Source: CAD feature listing. Evaluate the final solid. Frame: model axes, mm. Coordinates: 2 decimals unless noted, no trailing zeros. Order: outer loops, then holes, each group sorted by start corner. A loop starts at its lowest first (then second) coordinate and runs counter-clockwise, first axis right, second up.
Item 1: Ray query, line 1 (Y direction, x = 0, z = 3.6); line 2 (X direction, y = 67.5, z = 0.2); line 3 (X direction, y = -4.5, z = 2.15). Return the intervals inside material, ascending.
Item 2: Section D-D on z = 3.3. Return the cut outline in (x, y).
Item 3: Section B-B on x = -50. Return the cut outline in (y, z).
Item 4: Section A-A on y = 27.6. Return the cut outline in (x, z), then the cut area to 3 significant figures.
Item 5: Section C-C on x = 0. Return the cut outline in (y, z).
Item 6: Contact query for flat-ended pins moving along their axis: P1, Ø4, axis at x = 0, y = 27.6, coming from the +Z side; P2, Ø1.5, axis at y = 45.5, z = 2.5, coming from the -X side; P3, Ø2.5, axis at y = 9.5, z = 2, coming from the +X side. Output: stop coordinate, or through.
from build123d import *

# Parameters (mm, degrees)
SKETCH1_W           = 20
SKETCH1_H           = 160
SKETCH1_H_2         = 40
SKETCH1_W_2         = 70
BOSS_EXTRUDE1_DEPTH = 5
SKETCH2_R           = 2.25
CUT_EXTRUDE1_DEPTH  = 15


with BuildPart() as part:
    # Sketch1 → Boss-Extrude1 (new body)
    with BuildSketch(Plane.XY):
        with Locations((0, 20)):
            Rectangle(SKETCH1_W, SKETCH1_H)
        with Locations((0, -80)):
            Rectangle(SKETCH1_W, SKETCH1_H_2)
        with Locations((-45, -80)):
            Rectangle(SKETCH1_W_2, SKETCH1_H_2)
        with Locations((45, -80)):
            Rectangle(SKETCH1_W_2, SKETCH1_H_2)
    extrude(amount=BOSS_EXTRUDE1_DEPTH)

    # Sketch2 → Cut-Extrude1 (cut)
    with BuildSketch(Plane.XY.offset(5)):
        with Locations((0, -91.6)):
            Circle(SKETCH2_R)
        with Locations((-50, -76)):
            Circle(SKETCH2_R)
        with Locations((50, -76)):
            Circle(SKETCH2_R)
        with Locations((0, 27.6)):
            Circle(SKETCH2_R)
        with Locations((0, 67.6)):
            Circle(SKETCH2_R)
        with Locations((0, -32.4)):
            Circle(SKETCH2_R)
        with Locations((0, -61.6)):
            Circle(SKETCH2_R)
    extrude(amount=-CUT_EXTRUDE1_DEPTH, mode=Mode.SUBTRACT)


solid = part.part
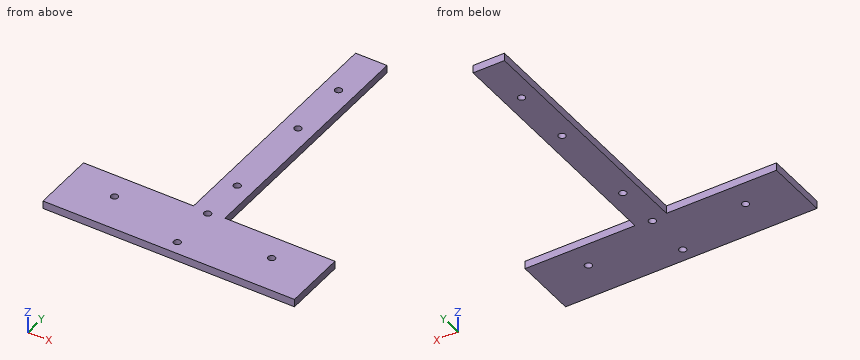
Answer list:
1. line 1: y = -100 to -93.85, -89.35 to -63.85, -59.35 to -34.65, -30.15 to 25.35, 29.85 to 65.35, 69.85 to 100
1. line 2: x = -10 to -2.25, 2.25 to 10
1. line 3: x = -10 to 10
2. outline: (-80, -100) - (80, -100) - (80, -60) - (10, -60) - (10, 100) - (-10, 100) - (-10, -60) - (-80, -60) - close; hole circle Ø4.5 at (-50, -76); hole circle Ø4.5 at (0, -91.6); hole circle Ø4.5 at (0, -61.6); hole circle Ø4.5 at (0, -32.4); hole circle Ø4.5 at (0, 27.6); hole circle Ø4.5 at (0, 67.6); hole circle Ø4.5 at (50, -76)
3. outline: (-100, 0) - (-78.25, 0) - (-78.25, 5) - (-100, 5) - close; (-73.75, 0) - (-60, 0) - (-60, 5) - (-73.75, 5) - close
4. outline: (-10, 0) - (-2.25, 0) - (-2.25, 5) - (-10, 5) - close; (2.25, 0) - (10, 0) - (10, 5) - (2.25, 5) - close
4. area: 77.5 mm2
5. outline: (-100, 0) - (-93.85, 0) - (-93.85, 5) - (-100, 5) - close; (-89.35, 0) - (-63.85, 0) - (-63.85, 5) - (-89.35, 5) - close; (-59.35, 0) - (-34.65, 0) - (-34.65, 5) - (-59.35, 5) - close; (-30.15, 0) - (25.35, 0) - (25.35, 5) - (-30.15, 5) - close; (29.85, 0) - (65.35, 0) - (65.35, 5) - (29.85, 5) - close; (69.85, 0) - (100, 0) - (100, 5) - (69.85, 5) - close
6. P1: passes through
6. P2: stops at x = -10
6. P3: stops at x = 10
